```python
from build123d import *

# Parameters (mm, degrees)
SKETCH1_W           = 75.947601036
SKETCH1_H           = 54.14073695
BOSS_EXTRUDE1_DEPTH = 1.778
SKETCH2_W           = 55.627601036
SKETCH2_H           = 33.82073695
SKETCH2_W_2         = 50.547601036
SKETCH2_H_2         = 28.74073695
EXTRUDE_THIN1_DEPTH = 17.78


with BuildPart() as part:
    # Sketch1 → Boss-Extrude1 (new body)
    with BuildSketch(Plane(origin=(0, 0, 0), x_dir=(1, 0, 0), z_dir=(0, 1, 0))):
        Rectangle(SKETCH1_W, SKETCH1_H)
    extrude(amount=BOSS_EXTRUDE1_DEPTH)

    # Sketch2 → Extrude-Thin1 (add)
    with BuildSketch(Plane(origin=(0, 1.778, 0), x_dir=(1, 0, 0), z_dir=(0, 1, 0))):
        Rectangle(SKETCH2_W, SKETCH2_H)
        Rectangle(SKETCH2_W_2, SKETCH2_H_2, mode=Mode.SUBTRACT)
    extrude(amount=EXTRUDE_THIN1_DEPTH)


solid = part.part
```
Read the model definition and answer for the solid it produces. Units are mm, in the model's axes. A direction names the side the tool comes from. Round coordinates to 2 decimals unless told otherwise and drop trailing zeros. Loops run counter-clockwise (first coordinate to the right, second up) from the corner with the lowest first, then second, coordinate; pieces in that order, holes last. Notation, with made-up numbers: (64.25, 3) -> (86.25, 3) arc R29 cw to (86.25, 23) -> close; hole circle Ø11 at (0.5, -4). An arc over 180 degrees is marked (long way). One line per item, written item: value.
1) Consider L1, parallel to Z at x = 15.5, y = 11.5; L2, parallel to X at y = 3.5, z = -3.5; L3, parallel to Y at x = -16.5, z = -3. Determine where each line is inside the solid, lowest interval first. Write a range as [from, to].
Answer list:
L1: z = [-16.91, -14.37], [14.37, 16.91]
L2: x = [-27.81, -25.27], [25.27, 27.81]
L3: y = [0, 1.78]
2) Flat-ended cylindrical pins translate along their axes: P1, Ø9, axis at x = 12, y = 7.5, coming from the +Z side; P2, Ø9, axis at x = -2.5, y = 14.5, coming from the -Z side; P3, Ø6, axis at x = 9.5, z = -6, coming from the -Y side; P4, Ø1.5, axis at y = 13, z = 0, coming from the -X side. Find the tip coordinate at first contact, or state that the pin passes through.
Answer list:
P1: stops at z = 16.91
P2: stops at z = -16.91
P3: stops at y = 0
P4: stops at x = -27.81
3) A cutting plane is placed at A-A (x = -11). Determine the outline of the cut face in (y, z).
Answer list:
outline: (0, -27.07) -> (1.78, -27.07) -> (1.78, -16.91) -> (19.56, -16.91) -> (19.56, -14.37) -> (1.78, -14.37) -> (1.78, 14.37) -> (19.56, 14.37) -> (19.56, 16.91) -> (1.78, 16.91) -> (1.78, 27.07) -> (0, 27.07) -> close
4) For faces 1 (the face through (27.814, 11, 0)), 2 (the face through (0, 1.778, 0)), 3 (the face through (-27.814, 11, 0)), determine the directions among +Z, -Z, +X, -X, +Y, -Y from which every point of the face is accessible in a straight line to the end or side of a thin tool.
Answer list:
face 1: +Z, -Z, +X, +Y
face 2: +Y
face 3: +Z, -Z, -X, +Y
5) The mould has two halves that part along Z. Classify faces 4 (the face through (-1, 1.778, -18)), 5 (the face through (0, 11, 16.91)), 6 (the face through (0, 11, -14.37)): pulls with the +Z half, pulls with the -Z half, needs draft (parallel to the pull), parting line crosses it, or undercut.
Answer list:
face 4: needs draft
face 5: pulls with the +Z half
face 6: undercut
6) A cutting plane is placed at D-D (x = -26.5). Determine the outline of the cut face in (y, z), and give its area (3 significant figures).
Answer list:
outline: (0, -27.07) -> (1.78, -27.07) -> (1.78, -16.91) -> (19.56, -16.91) -> (19.56, 16.91) -> (1.78, 16.91) -> (1.78, 27.07) -> (0, 27.07) -> close
area: 698 mm²
7) A cutting plane is placed at B-B (y = 12). Determine the outline of the cut face in (x, z), and give its area (3 significant figures).
Answer list:
outline: (-27.81, -16.91) -> (27.81, -16.91) -> (27.81, 16.91) -> (-27.81, 16.91) -> close; hole (-25.27, -14.37) -> (25.27, -14.37) -> (25.27, 14.37) -> (-25.27, 14.37) -> close
area: 429 mm²
8) A cutting plane is placed at C-C (z = -16). Determine the outline of the cut face in (x, y).
Answer list:
outline: (-37.97, 0) -> (37.97, 0) -> (37.97, 1.78) -> (27.81, 1.78) -> (27.81, 19.56) -> (-27.81, 19.56) -> (-27.81, 1.78) -> (-37.97, 1.78) -> close
